Can you work these out from the model? Positions are in its coordinate system, mm. A direction names the side the tool comes from. Coordinates: 2 decimals unless noted, no trailing zeros. Loops run counter-clockwise (first coordinate to the right, second up) from the corner with the lowest first, then second, coordinate; pieces in that order, holes last. Notation, with made-up numbers: M 73,-25 L 109,-25 A19 ccw 109,8 Z; hole C 61,56 d3. An arc over 180 degrees is marked long. Return JSON: item names as keys, results as strings. Group by question number.
```python
from build123d import *

# Parameters (mm, degrees)
BOSS_EXTRUDE1_DEPTH      = 3.175
M6_CLEARANCE_HOLE1_D     = 6.6
M6_CLEARANCE_HOLE1_DEPTH = 3.302
M6_CLEARANCE_HOLE1_TIP   = 1.982840043


with BuildPart() as part:
    # Sketch1 → Boss-Extrude1 (new body)
    with BuildSketch(Plane.XY):
        with BuildLine():
            Line((-79.409543338, -48.870574021), (-79.409543338, -29.820574021))
            Line((-79.409543338, -29.820574021), (-76.234543338, -29.820574021))
            Line((-76.234543338, -29.820574021), (-76.234543338, -24.740574021))
            Line((-76.234543338, -24.740574021), (-67.852543338, -24.740574021))
            ThreePointArc((-67.852543338, -24.740574021), (-64.175656813, -25.348124877), (-60.889653149, -27.10618986))
            Line((-60.889653149, -27.10618986), (-41.938948425, -46.672019211))
            ThreePointArc((-41.938948425, -46.672019211), (-41.391943029, -62.336204271), (-56.723167431, -65.594956616))
            Line((-56.723167431, -65.594956616), (-76.234543338, -55.220574021))
            Line((-76.234543338, -55.220574021), (-76.234543338, -48.870574021))
            Line((-76.234543338, -48.870574021), (-79.409543338, -48.870574021))
        make_face()
    extrude(amount=BOSS_EXTRUDE1_DEPTH)

    # M6 Clearance Hole1
    with Locations(Plane(origin=(0, 0, 0), x_dir=(-1, 0, 0), z_dir=(0, 0, -1))):
        with Locations((50.999370137, -54.830059564)):
            Hole(M6_CLEARANCE_HOLE1_D / 2, depth=M6_CLEARANCE_HOLE1_DEPTH)
            with Locations((0, 0, -(M6_CLEARANCE_HOLE1_DEPTH + M6_CLEARANCE_HOLE1_TIP / 2))):  # 118° drill point
                Cone(0, M6_CLEARANCE_HOLE1_D / 2, M6_CLEARANCE_HOLE1_TIP, mode=Mode.SUBTRACT)


solid = part.part
```
1) If we mould it in two halves opening along X, with no side actions, what happens to faces 4 (the face through (-51.5, -36.8, 1.6)), 5 (the face through (-41.25, -62.15, 1.57)), 6 (the face through (-51.715, -58.052, 1.61)), 7 (the face through (-78, -48.871, 2))? For each: +X half, -X half, draft (parallel to the pull), parting line (faces both ways), or undercut.
2) For pin 1 (1 mm diameter, centred on x = -78, z = 1, fed in from +Y); pin 2 (1.5 mm diameter, centred on y = -51, z = 2, fed in from +X); pin 3 (1.6 mm diameter, centred on y = -52.5, z = 2, fed in from -X), each with a flat end and sliding along its axis, tell me the tip position at first contact or that it passes through.
3) If I drill on line 1 (Y direction, x = -51.5, z = 2.2); line 2 (Y direction, x = -77, z = 1.6); line 3 (Y direction, x = -75, z = 1.35), over which ranges is the centre line in solid material (lowest first)? Write a range as from..to.
4) Suppose I cut it at D-D, the plane y = -28. List the corners of the cut face in (x, z) for me (3 decimals), then the cut area to 3 significant figures.
5) For faces 1 (the face through (-59, -46, 3.175)), 2 (the face through (-76.235, -52, 2)), 3 (the face through (-76.235, -27, 2)), which set-ups out of +Z, -Z, +X, -X, +Y, -Y let a thin tool reach every point of the face, with its end or its side?
6) Suppose I cut it at B-B, the plane y = -53. List the corners of the cut face in (x, z) for me (1 decimal).
7) Suppose I cut it at A-A, the plane z = 2.5. List the corners of the cut face in (x, y) for me.
8) Suppose I cut it at C-C, the plane x = -53.5. List the corners of the cut face in (y, z) for me (3 decimals), then the cut area to 3 significant figures.
Returned:
{
 "1": {"face 4": "+X half", "face 5": "parting line", "face 6": "undercut", "face 7": "draft"},
 "2": {"pin 1": "stops at y = -29.82", "pin 2": "stops at x = -39.2", "pin 3": "stops at x = -76.23"},
 "3": {"line 1": "y = -67.01..-58.09, -51.57..-36.8", "line 2": "y = -48.87..-29.82", "line 3": "y = -55.88..-24.74"},
 "4": {"outline": "M -76.235,0 L -60.024,0 L -60.024,3.175 L -76.235,3.175 Z", "area": "51.5 mm²"},
 "5": {"face 1": "+Z, +X, -X, +Y, -Y", "face 2": "+Z, -Z, -X, -Y", "face 3": "+Z, -Z, -X, +Y"},
 "6": {"outline": "M -76.2,0 L -53.7,0 L -53.7,3.2 L -76.2,3.2 Z; M -48.3,0 L -38.9,0 L -38.9,3.2 L -48.3,3.2 Z"},
 "7": {"outline": "M -79.41,-48.87 L -76.23,-48.87 L -76.23,-55.22 L -56.72,-65.59 A12.19 ccw -41.94,-46.67 L -60.89,-27.11 A11.43 ccw -67.85,-24.74 L -76.23,-24.74 L -76.23,-29.82 L -79.41,-29.82 Z; hole C -51,-54.83 d6.6"},
 "8": {"outline": "M -66.763,0 L -56.983,0 L -56.983,3.175 L -66.763,3.175 Z; M -52.677,0 L -34.736,0 L -34.736,3.175 L -52.677,3.175 Z", "area": "88.0 mm²"}
}
